Can you work these out from the model? Positions are in its coordinate system, mm. A direction names the side the tool comes from. Coordinates: 2 decimals unless noted, no trailing zeros. Order: outer loops, then holes, each group sorted by start corner. A loop starts at its lowest first (then second) coordinate and runs counter-clockwise, first axis right, second up. Notation, with made-up numbers: (-32, 75.5) -> (-12, 75.5) arc R29 cw to (-12, 100.5) -> close; hole circle Ø6 at (85, 34). An arc over 180 degrees is marked (long way). Use a Markdown table: item, result. Add a question column.
1. For faces 4 (the flat face through (0, 3, 0)), 5 (the flat face through (8, 4, 1)), 6 (the flat face through (9.6, 0, 1)), which set-ups out of +Z, -Z, +X, -X, +Y, -Y let a thin tool reach every point of the face, with its end or its side?
2. Suppose I cut it at C-C, the plane z = 0.7. List the corners of the cut face in (x, y) for me.
3. Suppose I cut it at D-D, the plane x = -1.25. List the corners of the cut face in (y, z) for me, then the cut area to 3 significant figures.
4. If I drill on line 1 along Y through (x, z) = (-8, 0.8); line 2 along X through (y, z) = (0.5, 0.6); line 3 along Y through (x, z) = (-0.25, 1.75), over which ranges is the centre line in solid material (lowest first)? Write a range as from..to.
5. We'd pull the mould along X, two halves only. Please class faces 1 (the flat face through (-2.2, 7.5, 1)), 2 (the flat face through (-4.4, 0, 1)), 3 (the flat face through (-8, 4, 1)): pulls with the +X half, pulls with the -X half, needs draft (parallel to the pull), parting line crosses it, or undercut.
6. Suppose I cut it at A-A, the plane y = 0. List the corners of the cut face in (x, z) for me, then the cut area to 3 significant figures.
7. For pin 1 Ø0.6 at (x, z) = (7, 1) entering from +Y; pin 2 Ø1 at (x, z) = (4, 1.5) entering from +Y, each with a flat end and sliding along its axis, tell me the tip position at first contact or that it passes through.
8. Suppose I cut it at B-B, the plane x = -8.25. List the corners of the cut face in (y, z) for me.
```python
from build123d import *

# Parameters (mm, degrees)
SKETCH_1_R      = 1.5
SKETCH_1_W      = 5.2
SKETCH_1_H      = 2.2
EXTRUDE_1_DEPTH = 2


with BuildPart() as part:
    # 草图1 → 凸台-拉伸1 (new body)
    with BuildSketch(Plane.XY):
        Polygon((-11, 0), (-11, -3), (11, -3), (11, 0), (11, 4), (4.4, 4), (0, 11), (-4.4, 4), (-11, 4), align=None)
        Circle(SKETCH_1_R, mode=Mode.SUBTRACT)
        with Locations((7, 0)):
            Rectangle(SKETCH_1_W, SKETCH_1_H, mode=Mode.SUBTRACT)
        with Locations((-7, 0)):
            Rectangle(SKETCH_1_W, SKETCH_1_H, mode=Mode.SUBTRACT)
    extrude(amount=EXTRUDE_1_DEPTH)


solid = part.part
```
Worked out:
| question | item | result |
|---|---|---|
| 1 | face 4 | -Z, +X, -X, +Y, -Y |
| 1 | face 5 | +Z, -Z, +X, +Y |
| 1 | face 6 | +Z, -Z |
| 2 | outline | (-11, -3) -> (11, -3) -> (11, 4) -> (4.4, 4) -> (0, 11) -> (-4.4, 4) -> (-11, 4) -> close; hole (-9.6, -1.1) -> (-4.4, -1.1) -> (-4.4, 1.1) -> (-9.6, 1.1) -> close; hole circle Ø3 at (0, 0); hole (4.4, -1.1) -> (9.6, -1.1) -> (9.6, 1.1) -> (4.4, 1.1) -> close |
| 3 | outline | (-3, 0) -> (-0.83, 0) -> (-0.83, 2) -> (-3, 2) -> close; (0.83, 0) -> (9.01, 0) -> (9.01, 2) -> (0.83, 2) -> close |
| 3 | area | 20.7 mm² |
| 4 | line 1 | y = -3..-1.1, 1.1..4 |
| 4 | line 2 | x = -11..-9.6, -4.4..-1.41, 1.41..4.4, 9.6..11 |
| 4 | line 3 | y = -3..-1.48, 1.48..10.6 |
| 5 | face 1 | pulls with the -X half |
| 5 | face 2 | undercut |
| 5 | face 3 | needs draft |
| 6 | outline | (-11, 0) -> (-9.6, 0) -> (-9.6, 2) -> (-11, 2) -> close; (-4.4, 0) -> (-1.5, 0) -> (-1.5, 2) -> (-4.4, 2) -> close; (1.5, 0) -> (4.4, 0) -> (4.4, 2) -> (1.5, 2) -> close; (9.6, 0) -> (11, 0) -> (11, 2) -> (9.6, 2) -> close |
| 6 | area | 17.2 mm² |
| 7 | pin 1 | stops at y = 4 |
| 7 | pin 2 | stops at y = 5.43 |
| 8 | outline | (-3, 0) -> (-1.1, 0) -> (-1.1, 2) -> (-3, 2) -> close; (1.1, 0) -> (4, 0) -> (4, 2) -> (1.1, 2) -> close |
